For this review, take the finished solid that the model builds, in its own axes (mm). Face numbers are marked on the shaded views. A direction names the side the tool comes from. Give positions to 0.01 mm unless a question says otherwise; leave off trailing zeros. Loops run counter-clockwise (first coordinate to the right, second up) from the corner with the lowest first, then second, coordinate; pieces in that order, holes last. Notation, with made-up numbers: (-17.5, 87) - (10.5, 87) arc R11 ccw to (10.5, 92) - close; hole circle Ø1 at (-13.5, 83). An arc over 180 degrees is marked (long way). Put each result on its own line as item: value.
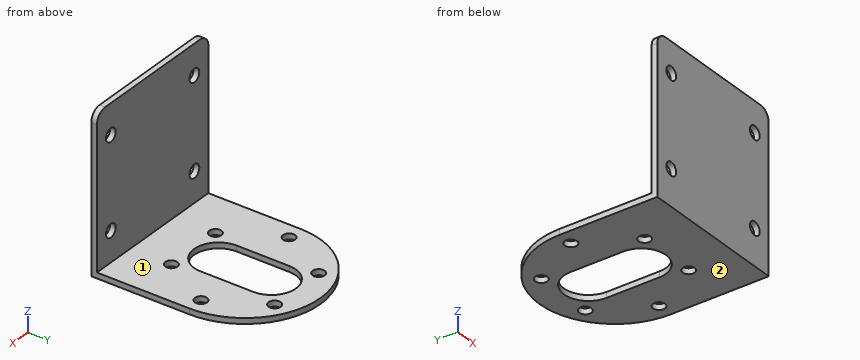
from build123d import *

# Parameters (mm, degrees)
SKETCH1_W           = 40
SKETCH1_H           = 40
SKETCH1_R           = 1.75
BOSS_EXTRUDE1_DEPTH = 1.5
FILLET1_R           = 3
SKETCH2_R           = 1.6
BOSS_EXTRUDE2_DEPTH = 1.5


with BuildPart() as part:
    # Sketch1 → Boss-Extrude1 (new body)
    with BuildSketch(Plane(origin=(0, 0, 0), x_dir=(1, 0, 0), z_dir=(0, 1, 0))):
        Rectangle(SKETCH1_W, SKETCH1_H)
        with Locations((-15, -12)):
            Circle(SKETCH1_R, mode=Mode.SUBTRACT)
        with Locations((15, -12)):
            Circle(SKETCH1_R, mode=Mode.SUBTRACT)
        with Locations((15, 12)):
            Circle(SKETCH1_R, mode=Mode.SUBTRACT)
        with Locations((-15, 12)):
            Circle(SKETCH1_R, mode=Mode.SUBTRACT)
    extrude(amount=BOSS_EXTRUDE1_DEPTH)

    # Fillet1
    fillet1_edges = [part.edges().sort_by_distance(p)[0] for p in [
        (20, 0.75, 20),
        (-20, 0.75, 20),
    ]]
    fillet(fillet1_edges, radius=FILLET1_R)

    # Sketch2 → Boss-Extrude2 (add)
    with BuildSketch(Plane(origin=(0, 0, -20), x_dir=(-1, 0, 0), z_dir=(0, 0, -1))):
        with BuildLine():
            Line((-20, 0), (20, 0))
            Line((20, 0), (20, 26))
            ThreePointArc((20, 26), (0, 46), (-20, 26))
            Line((-20, 26), (-20, 0))
        make_face()
        with Locations((15.81171166, 26)):
            Circle(SKETCH2_R, mode=Mode.SUBTRACT)
        with Locations((7.90585583, 12.306656025)):
            Circle(SKETCH2_R, mode=Mode.SUBTRACT)
        with Locations((-7.90585583, 12.306656025)):
            Circle(SKETCH2_R, mode=Mode.SUBTRACT)
        with Locations((-15.81171166, 26)):
            Circle(SKETCH2_R, mode=Mode.SUBTRACT)
        with Locations((-7.90585583, 39.693343975)):
            Circle(SKETCH2_R, mode=Mode.SUBTRACT)
        with Locations((7.90585583, 39.693343975)):
            Circle(SKETCH2_R, mode=Mode.SUBTRACT)
        with BuildLine():
            Line((-6.5, 33), (-6.5, 19))
            ThreePointArc((-6.5, 19), (0, 12.5), (6.5, 19))
            Line((6.5, 19), (6.5, 33))
            ThreePointArc((6.5, 33), (0, 39.5), (-6.5, 33))
        make_face(mode=Mode.SUBTRACT)
    extrude(amount=BOSS_EXTRUDE2_DEPTH)


solid = part.part
1) Take a section at B-B on y = 29. State the section outline as (x, z) points.
Geometry check:
outline: (-19.77, -21.5) - (-6.5, -21.5) - (-6.5, -20) - (-19.77, -20) - close; (6.5, -21.5) - (19.77, -21.5) - (19.77, -20) - (6.5, -20) - close
2) Take a section at C-C on x = 0.5. State the section outline as (y, z) points.
Geometry check:
outline: (0, -21.5) - (12.52, -21.5) - (12.52, -20) - (1.5, -20) - (1.5, 20) - (0, 20) - close; (39.48, -21.5) - (45.99, -21.5) - (45.99, -20) - (39.48, -20) - close
3) For the marked faces 1 and 2, list the 3-axis set-ups (+Z, -Z, +X, -X, +Y, -Y) from which the entire face can be reached by the end or side of a thin tool; tool diameter is ignored.
Geometry check:
face 1: +Z, +X, -X, +Y
face 2: -Z, +X, -X, +Y, -Y
4) Wall thickness on line 1 (X direction, y = 0.55, z = -12); line 2 (Y direction, x = 4.5, z = 14); line 3 (Z direction, x = -10.5, y = 31): over which ranges is each line inside the solid? List them lowest first.
Geometry check:
line 1: x = -20 to -16.75, -13.25 to 13.25, 16.75 to 20
line 2: y = 0 to 1.5
line 3: z = -21.5 to -20
5) Take a section at A-A on z = 12. State the section outline as (x, y) points, and give its area (3 significant figures).
Geometry check:
outline: (-20, 0) - (-16.75, 0) - (-16.75, 1.5) - (-20, 1.5) - close; (-13.25, 0) - (13.25, 0) - (13.25, 1.5) - (-13.25, 1.5) - close; (16.75, 0) - (20, 0) - (20, 1.5) - (16.75, 1.5) - close
area: 49.5 mm²
6) Insertion check: pin 1 Ø5.5 at (x, z) = (-15, 12) entering from +Y; pin 2 Ø4 at (x, y) = (7.91, 39.69) entering from +Z. Each pin has a flat end and moves straight along its axis. Give the tip position at first contact, or say it passes through.
Geometry check:
pin 1: stops at y = 1.5
pin 2: stops at z = -20
7) Take a section at D-D on x = -12. State the section outline as (y, z) points, and give its area (3 significant figures).
Geometry check:
outline: (0, -21.5) - (42, -21.5) - (42, -20) - (1.5, -20) - (1.5, 20) - (0, 20) - close
area: 123 mm²
